Verification items for the finished model (mm, model axes). A direction names the side the tool comes from. Round coordinates to 2 decimals unless told otherwise and drop trailing zeros. Write each loop counter-clockwise with the first axis right and the second up, starting at its lowest first coordinate (ties: lowest second). Pieces come first, ordered by that corner, then holes. Notation, with made-up numbers: (-33, 32) -> (-25, 32) arc R23 ccw to (-25, 56) -> close; hole circle Ø4 at (-12, 68.25). An arc over 180 degrees is marked (long way). Answer as a JSON object with one key per item and string values. Group by question number.
(1) Sectioned sample at D-D on z = 4. Count the separate pieces of the cut face and the enclosed holes in it, and give its area (3 significant figures).
(2) Scan lines: L1, parallel to Y at x = 23, z = 9.25; L2, parallel to Y at x = -23, z = 12.25; L3, parallel to X at y = 124, z = 5. Record each from-to range of solid material in increasing order. Write a range as from..to.
(3) Sectioned sample at B-B on z = -10. Record the cut outline in (x, y).
(4) Gauge pin test, flat ends, axial feed: pin 1 Ø5 at (x, y) = (-23.5, 79.5) entering from +Z; pin 2 Ø8 at (y, z) = (-32.5, 8.5) entering from -X; pin 3 Ø8 at (x, y) = (20, 90.5) entering from -Z. Record the tip position at first contact, or that the pin passes through.
(5) Sectioned sample at C-C on y = 20. Record the cut outline in (x, z), and give its area (3 significant figures).
(6) Set-up check for faces 4 (the face through (-33, 12.5, 15)), 5 (the face through (0, 51, 0)), 6 (the face through (-30, -23, 10)): record each of +Z, -Z, +X, -X, +Y, -Y from which the full face is reachable in a straight line by a thin tool's end or side.
(7) Draft check along Y on faces 1 (the face through (1, 139.5, 2)), 2 (the face through (-20, 93, 6)), 3 (the face through (30, 79, -10)). Enter one of: released by +Y, released by -Y, zero draft, split by the parting line, or undercut.
(8) Sectioned sample at A-A on y = -6.5. Record the cut outline in (x, z).
```python
from build123d import *

# Parameters (mm, degrees)
SKETCH_W        = 60
SKETCH_H        = 25
SKETCH_R        = 3.3
PAD_DEPTH       = 25.9
SKETCH001_W     = 60
SKETCH001_H     = 11.1
PAD001_DEPTH    = 127
SKETCH002_R     = 2.5
POCKET_DEPTH    = 11.101
PAD002_DEPTH    = 60
SKETCH004_W     = 152
SKETCH004_H     = 32.1
PAD003_DEPTH    = 10
SKETCH005_W     = 152
SKETCH005_H     = 32.1
PAD004_DEPTH    = 10
PAD005_DEPTH    = 25
SKETCH007_W     = 50
SKETCH007_H     = 18
POCKET001_DEPTH = 10
POCKET002_DEPTH = 10
SKETCH009_W     = 60
SKETCH009_H     = 15
PAD006_DEPTH    = 27
PAD007_DEPTH    = 60


with BuildPart() as part:
    # Sketch → Pad (new body)
    with BuildSketch(Plane.XY):
        Rectangle(SKETCH_W, SKETCH_H)
        with Locations((-23, 6.5)):
            Circle(SKETCH_R, mode=Mode.SUBTRACT)
        with Locations((-23, -6.5)):
            Circle(SKETCH_R, mode=Mode.SUBTRACT)
        with Locations((23, -6.5)):
            Circle(SKETCH_R, mode=Mode.SUBTRACT)
        with Locations((23, 6.5)):
            Circle(SKETCH_R, mode=Mode.SUBTRACT)
    extrude(amount=PAD_DEPTH)

    # Sketch001 (on Face1 of Pad) → Pad001 (join)
    with BuildSketch(Plane(origin=(0, 12.5, 0), x_dir=(-1, 0, 0), z_dir=(0, 1, 0))):
        with Locations((0, 5.55)):
            Rectangle(SKETCH001_W, SKETCH001_H)
    extrude(amount=PAD001_DEPTH)

    # Sketch002 (on Face2 of Pad001) → Pocket (cut, through all)
    with BuildSketch(Plane.XY.offset(11.1)):
        with Locations((-20, 124.5)):
            Circle(SKETCH002_R)
        with Locations((20, 124.5)):
            Circle(SKETCH002_R)
        with Locations((-20, 90.5)):
            Circle(SKETCH002_R)
        with Locations((20, 90.5)):
            Circle(SKETCH002_R)
    extrude(amount=-POCKET_DEPTH, mode=Mode.SUBTRACT)

    # Sketch003 (on Face6 of Pocket) → Pad002 (join)
    with BuildSketch(Plane.YZ.offset(30)):
        Polygon((12.5, 25.9), (32.5, 11.1), (12.5, 0), align=None)
    extrude(amount=-PAD002_DEPTH)

    # Sketch004 (on Face7 of Pad002) → Pad003 (join)
    with BuildSketch(Plane.YZ.offset(30)):
        with Locations((63.5, -4.95)):
            Rectangle(SKETCH004_W, SKETCH004_H)
    extrude(amount=PAD003_DEPTH)

    # Sketch005 (on Face20 of Pad003) → Pad004 (join)
    with BuildSketch(Plane(origin=(-30, 0, 0), x_dir=(0, -1, 0), z_dir=(-1, 0, 0))):
        with Locations((-63.5, -4.95)):
            Rectangle(SKETCH005_W, SKETCH005_H)
    extrude(amount=PAD004_DEPTH)

    # Sketch006 (on Face3 of Pad004) → Pad005 (join)
    with BuildSketch(Plane.XZ.offset(12.5)):
        Polygon((40, 11.1), (30, 11.1), (30, 25.9), align=None)
        Polygon((-30, 25.9), (-30, 11.1), (-40, 11.1), align=None)
    extrude(amount=-PAD005_DEPTH)

    # Sketch007 (on Face5 of Pad005) → Pocket001 (cut)
    with BuildSketch(Plane.YZ.offset(40)):
        with Locations((41.5, -12)):
            Rectangle(SKETCH007_W, SKETCH007_H)
    extrude(amount=-POCKET001_DEPTH, mode=Mode.SUBTRACT)

    # Sketch008 (on Face25 of Pocket001) → Pocket002 (cut)
    with BuildSketch(Plane(origin=(-40, 0, 0), x_dir=(0, -1, 0), z_dir=(-1, 0, 0))):
        with BuildLine():
            ThreePointArc((-31.5, -21), (-41.297959, -13), (-51.095918, -21))
            Line((-51.095918, -21), (-31.5, -21))
        make_face()
    extrude(amount=-POCKET002_DEPTH, mode=Mode.SUBTRACT)

    # Sketch009 (on Face29 of Pocket002) → Pad006 (join)
    with BuildSketch(Plane.XZ.offset(12.5)):
        with Locations((0, 7.5)):
            Rectangle(SKETCH009_W, SKETCH009_H)
    extrude(amount=PAD006_DEPTH)

    # Sketch010 (on Face29 of Pad006) → Pad007 (join)
    with BuildSketch(Plane.YZ.offset(30)):
        Polygon((-32.5, 15), (-12.5, 15), (-12.5, 25.9), align=None)
    extrude(amount=-PAD007_DEPTH)


solid = part.part
```
Computed values:
{
 "1": {"separate pieces": "1", "enclosed holes": "8", "area": "13,600 mm2"},
 "2": {"L1": "-39.5..-9.8, -3.2..3.2, 9.8..139.5", "L2": "-39.5..-9.8, -3.2..3.2, 9.8..30.95", "L3": "-40..-22.45, -17.55..17.55, 22.45..40"},
 "3": {"outline": "(-40, -12.5) -> (-30, -12.5) -> (-30, 139.5) -> (-40, 139.5) -> close; (30, -12.5) -> (40, -12.5) -> (40, 16.5) -> (30, 16.5) -> close; (30, 66.5) -> (40, 66.5) -> (40, 139.5) -> (30, 139.5) -> close"},
 "4": {"pin 1": "z = 11.1", "pin 2": "x = -30", "pin 3": "z = 0"},
 "5": {"outline": "(-40, -21) -> (-30, -21) -> (-30, 0) -> (30, 0) -> (30, -3) -> (40, -3) -> (40, 11.1) -> (30, 11.1) -> (30, 20.35) -> (-30, 20.35) -> (-30, 11.1) -> (-40, 11.1) -> close", "area": "1,680 mm2"},
 "6": {"face 4": "+Z, -X, +Y", "face 5": "-Z, +Y, -Y", "face 6": "+Z, -Z, -X, -Y"},
 "7": {"face 1": "released by +Y", "face 2": "undercut", "face 3": "zero draft"},
 "8": {"outline": "(-40, -21) -> (-30, -21) -> (-30, 0) -> (-26.3, 0) -> (-26.3, 25.9) -> (-30, 25.9) -> (-40, 11.1) -> close; (-19.7, 0) -> (19.7, 0) -> (19.7, 25.9) -> (-19.7, 25.9) -> close; (26.3, 0) -> (30, 0) -> (30, -21) -> (40, -21) -> (40, 11.1) -> (30, 25.9) -> (26.3, 25.9) -> close"}
}
